CAD build for the part. Positions are in the model's coordinates, mm. Face numbers are marked on the shaded views. A direction names the side the tool comes from. Coordinates: 2 decimals unless noted, no trailing zeros. Order: outer loops, then holes, each group sorted by start corner. A loop starts at its lowest first (then second) coordinate and runs counter-clockwise, first axis right, second up. Notation, with made-up numbers: M 75,5.5 L 103,5.5 A26 cw 103,29.5 Z; hole C 84.5,1.25 d4. An arc over 180 degrees is marked long. One line per item, written item: value.
from build123d import *

# Parameters (mm, degrees)
ESQUISSE1_W                  = 80
ESQUISSE1_H                  = 30
BOSS_EXTRU_1_DEPTH           = 5
ENL_V_MAT_EXTRU_1_DEPTH      = 86.586213843
ENL_V_MAT_EXTRU_1_DEPTH_BACK = 86.586213843
ESQUISSE2_R                  = 3.25
ESQUISSE2_R_2                = 3
CONG_1_R                     = 5
BOSS_EXTRU_2_DEPTH           = 5


with BuildPart() as part:
    # Esquisse1 → Boss.-Extru.1 (new body)
    with BuildSketch(Plane.XY):
        with Locations((40, 15)):
            Rectangle(ESQUISSE1_W, ESQUISSE1_H)
    extrude(amount=BOSS_EXTRU_1_DEPTH)

    # Esquisse2 → Enlèv. mat.-Extru.1 (cut, two sides: drawn at the far end of the back side and taken through both)
    with BuildSketch(Plane.XY.offset(5).offset(-ENL_V_MAT_EXTRU_1_DEPTH_BACK)):
        with Locations((15, 20)):
            Circle(ESQUISSE2_R)
        with Locations(Location((65, 20, 0), (0, 0, 180))):
            Circle(ESQUISSE2_R)
        with Locations((10, 7)):
            Circle(ESQUISSE2_R_2)
        with Locations(Location((70, 7, 0), (0, 0, 180))):
            Circle(ESQUISSE2_R_2)
    extrude(amount=ENL_V_MAT_EXTRU_1_DEPTH + ENL_V_MAT_EXTRU_1_DEPTH_BACK, mode=Mode.SUBTRACT)

    # Congé1
    cong_1_edges = [part.edges().sort_by_distance(p)[0] for p in [
        (0, 30, 2.5),
        (80, 30, 2.5),
        (80, 0, 2.5),
        (0, 0, 2.5),
    ]]
    fillet(cong_1_edges, radius=CONG_1_R)

    # Esquisse3 → Boss.-Extru.2 (add)
    with BuildSketch(Plane.XY.offset(5)):
        with BuildLine():
            Line((20.175853906, 30), (62.880368617, 30))
            add(Edge.make_bspline(
                [(62.880368617, 30), (56.248577834, 34.044178021), (43.342547907, 38.777474561), (30.753908623, 29.855151718), (23.756853958, 30.615618698), (20.175853906, 30)],
                knots=[0, 0, 0, 0, 0.562893367, 0.745092862, 1, 1, 1, 1], degree=3))
        make_face()
    extrude(amount=-BOSS_EXTRU_2_DEPTH)


solid = part.part
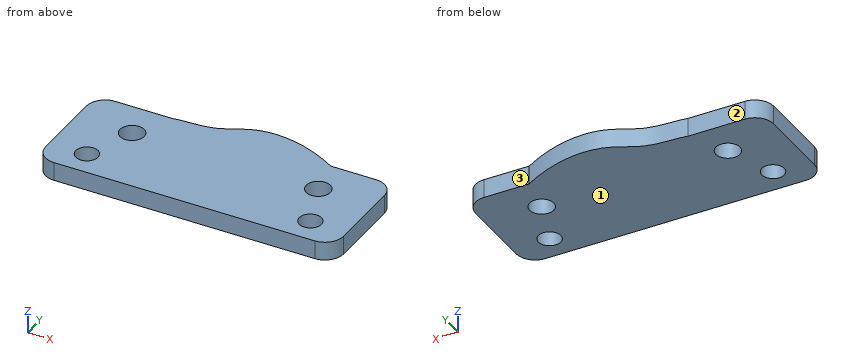
Q1. Slice it at D-D (x = 15). List the corners of the cut face in (y, z).
Recorded:
outline: M 0,0 L 16.75,0 L 16.75,5 L 0,5 Z; M 23.25,0 L 30,0 L 30,5 L 23.25,5 Z
Q2. Which spindle directions (+Z, -Z, +X, -X, +Y, -Y) get a long thin tool onto all of the face, cutting with end or side? Do the marked faces 1, 2 and 3. Say none if no direction does.
Recorded:
face 1: -Z, +X, -X, +Y, -Y
face 2: +Z, -Z, -X, +Y
face 3: +Z, -Z, +X, +Y
Q3. Slice it at B-B (x = 70). List the corners of the cut face in (y, z), plus the area to 3 significant figures.
Recorded:
outline: M 0,0 L 4,0 L 4,5 L 0,5 Z; M 10,0 L 30,0 L 30,5 L 10,5 Z
area: 120 mm^2
Q4. Slice it at C-C (y = 20). List the corners of the cut face in (x, z), plus the area to 3 significant figures.
Recorded:
outline: M 0,0 L 11.75,0 L 11.75,5 L 0,5 Z; M 18.25,0 L 61.75,0 L 61.75,5 L 18.25,5 Z; M 68.25,0 L 80,0 L 80,5 L 68.25,5 Z
area: 335 mm^2
Q5. Slice it at A-A (y = 7). List the corners of the cut face in (x, z).
Recorded:
outline: M 0,0 L 7,0 L 7,5 L 0,5 Z; M 13,0 L 67,0 L 67,5 L 13,5 Z; M 73,0 L 80,0 L 80,5 L 73,5 Z
Q6. Drill centre lines: line 1 along Y through (x, z) = (10, 3); line 2 along Y through (x, z) = (15, 1.95); line 3 along X through (y, z) = (18, 4.35). Where is each one in solid material? Low to high.
Recorded:
line 1: y = 0 to 4, 10 to 30
line 2: y = 0 to 16.75, 23.25 to 30
line 3: x = 0 to 12.44, 17.56 to 62.44, 67.56 to 80
